from build123d import *

# Parameters (mm, degrees)
SKETCH1_R           = 114.3
BOSS_EXTRUDE1_DEPTH = 6.35
SKETCH2_W           = 6.35
SKETCH2_H           = 114.3
CUT_EXTRUDE1_DEPTH  = 6.35
SKETCH3_W           = 127
SKETCH3_H           = 6.35
CUT_EXTRUDE2_DEPTH  = 162.769287876
SKETCH4_W           = 6.35
SKETCH4_H           = 63.5
CUT_EXTRUDE3_DEPTH  = 162.769287876


with BuildPart() as part:
    # Sketch1 → Boss-Extrude1 (new body)
    with BuildSketch(Plane(origin=(0, 0, 0), x_dir=(1, 0, 0), z_dir=(0, 1, 0))):
        with Locations(Location((0, 0, 0), (0, 0, 270))):
            Circle(SKETCH1_R)
    extrude(amount=BOSS_EXTRUDE1_DEPTH)

    # Sketch2 → Cut-Extrude1 (cut)
    with BuildSketch(Plane(origin=(0, 6.35, 0), x_dir=(1, 0, 0), z_dir=(0, 1, 0))):
        with Locations((0, -57.15)):
            Rectangle(SKETCH2_W, SKETCH2_H)
    extrude(amount=-CUT_EXTRUDE1_DEPTH, mode=Mode.SUBTRACT)

    # Sketch3 → Cut-Extrude2 (cut, through all)
    with BuildSketch(Plane(origin=(0, 6.35, 0), x_dir=(1, 0, 0), z_dir=(0, 1, 0))):
        Rectangle(SKETCH3_W, SKETCH3_H)
    extrude(amount=-CUT_EXTRUDE2_DEPTH, mode=Mode.SUBTRACT)

    # Sketch4 → Cut-Extrude3 (cut, through all)
    with BuildSketch(Plane(origin=(0, 6.35, 0), x_dir=(1, 0, 0), z_dir=(0, 1, 0))):
        with Locations((0, 31.75)):
            Rectangle(SKETCH4_W, SKETCH4_H)
    extrude(amount=-CUT_EXTRUDE3_DEPTH, mode=Mode.SUBTRACT)


solid = part.part
Input: part model. Units: mm. Frame: model coordinates. A direction names the side the tool comes from. Round coordinates to 2 decimals unless told otherwise and drop trailing zeros. Order: outer loops, then holes, each group sorted by start corner. A loop starts at its lowest first (then second) coordinate and runs counter-clockwise, first axis right, second up.
1. Mould query, pull axis X, two halves, no side actions, for faces 1 (the face through (-24, 6.35, 24)), 2 (the face through (4.98, 3.13, -114.19)), 3 (the face through (0, 3, -63.5)), 4 (the face through (3.175, 3, 59)). Classes: released by +X, released by -X, zero draft, split by the parting line, or undercut.
The answers:
face 1: zero draft
face 2: split by the parting line
face 3: undercut
face 4: undercut
2. Material intervals for line 1 (Z direction, x = -10, y = 0.5) (3 decimals); line 2 (X direction, y = 3.75, z = -3); line 3 (X direction, y = 1.25, z = -11.5) (3 decimals), sorted ascending.
The answers:
line 1: z = -113.862 to -3.175, 3.175 to 113.862
line 2: x = -114.26 to -63.5, 63.5 to 114.26
line 3: x = -113.72 to -3.175, 3.175 to 113.72
3. Cut plane B-B, the plane x = -57. Output: boundary loops of the cut face in (y, z) (3 decimals), then the cut area to 3 significant figures.
The answers:
outline: (0, -99.073) - (6.35, -99.073) - (6.35, -3.175) - (0, -3.175) - close; (0, 3.175) - (6.35, 3.175) - (6.35, 99.073) - (0, 99.073) - close
area: 1,220 mm2
4. Pin query (flat end, axial travel): P1, Ø1.9, axis at x = 0.5, y = 3.5, coming from the +Z side; P2, Ø3, axis at x = -37, y = 4.5, coming from the -Z side; P3, Ø3, axis at y = 3, z = -42, coming from the +X side. Return the tip coordinate at first contact, or that it passes through.
The answers:
P1: stops at z = -63.5
P2: stops at z = -108.65
P3: stops at x = 106.88
5. Cut plane C-C, the plane y = 3.25. Output: boundary loops of the cut face in (x, z) (3 decimals), then the cut area to 3 significant figures.
The answers:
outline: (-63.5, -3.175) - (-63.5, 3.175) - (-3.175, 3.175) - (-3.175, 114.256) arc R114.3 ccw (long way) to (3.175, 114.256) - (3.175, 3.175) - (63.5, 3.175) - (63.5, -3.175) - (3.175, -3.175) - (3.175, -63.5) - (-3.175, -63.5) - (-3.175, -3.175) - close
area: 39,100 mm2
6. Cut plane A-A, the plane z = 0. Output: boundary loops of the cut face in (x, y).
The answers:
outline: (-114.3, 0) - (-63.5, 0) - (-63.5, 6.35) - (-114.3, 6.35) - close; (63.5, 0) - (114.3, 0) - (114.3, 6.35) - (63.5, 6.35) - close
7. Cut plane D-D, the plane x = 0. Output: boundary loops of the cut face in (y, z).
The answers:
outline: (0, -114.3) - (6.35, -114.3) - (6.35, -63.5) - (0, -63.5) - close
8. Set-up query: faces 5 (the face through (-63.5, 3, 0)), 6 (the face through (-3.175, 3, 59)), 7 (the face through (-24, 0, 24)). Return all of +Z, -Z, +X, -X, +Y, -Y with unobstructed straight access to the full face (end or side cutting, diameter ignored); none if empty.
The answers:
face 5: +Y, -Y
face 6: +Z, +Y, -Y
face 7: +Z, -Z, +X, -X, -Y
